CAD build for the part. Positions are in the model's coordinates, mm. Face numbers are marked on the shaded views. A direction names the side the tool comes from. Coordinates: 2 decimals unless noted, no trailing zeros. Loops run counter-clockwise (first coordinate to the right, second up) from the corner with the lowest first, then second, coordinate; pieces in that order, holes last. Notation, with made-up numbers: (20.25, -10.75) -> (56.25, -10.75) arc R17 ccw to (56.25, 3.25) -> close; hole circle Ø8 at (-22.75, 62). An arc over 180 degrees is marked (long way). Return JSON: item names as keys, results as strings. Group by question number.
(1) Saw through at B-B on y = 10.5. Write the cut outline in (x, z).
(2) Saw through at C-C on y = 5.25. Write the cut outline in (x, z), then the cut area to 3 significant figures.
(3) Flat gauge pins, fed straight in: pin 1 Ø4 at (x, y) = (-2, 14.5) entering from +Z; pin 2 Ø1.6 at (x, z) = (0, 0) entering from +Y; pin 3 Ø5 at (x, z) = (-2, 1.5) entering from +Y; pin 4 Ø4 at (y, z) = (18.5, 7.5) entering from +X. Where does each tip first touch, or does it go through?
(4) Tool access for the marked faces 1, 2 and 3: list every direction of +Z, -Z, +X, -X, +Y, -Y with a clear straight run to the whole face (end or side of a thin tool).
(5) Saw through at A-A on z = 0. Write the cut outline in (x, y), then the cut area to 3 significant figures.
(6) Probe L1, parallel to Z at x = 0, y = 3.85; L2, parallel to Z at x = 0, y = 11.5; L3, parallel to X at y = 0.35, z = 0. List the from-to ranges inside material, lowest first.
Autodesk Fusion 360 part; units mm, degrees
sketch "Sketch1" plane through (0, 0, 0) normal (0, 0, 1) x (1, 0, 0)
  line L0 (0, 0) -> (-8, 0)
  line L1 (-8, 0) -> (-8, 19)
  line L2 (-8, 19) -> (0, 19)
  line L3 (0, 19) -> (0, 0)
  line L4 (0, 19) -> (-6.75, 19)
  line L5 (-6.75, 19) -> (-6.75, 7)
  line L6 (-6.75, 7) -> (0, 7)
  line L7 (0, 7) -> (0, 19)
  line L8 (0, 7) -> (-3.5, 7)
  line L9 (-3.5, 7) -> (-3.5, 1)
  line L10 (-3.5, 1) -> (0, 1)
  line L11 (0, 1) -> (0, 7)
  line L12 (0, 19) -> (-11, 19)
  line L13 (-11, 19) -> (-11, 21)
  line L14 (-11, 21) -> (0, 21)
  line L15 (0, 21) -> (0, 19)
  line L16 (-6.75, 19) -> (-6.75, 21)
  line L17 (0, 1) -> (-1, 1)
  line L18 (-1, 1) -> (-1, 0)
  line L19 (-1, 0) -> (0, 0)
  line L20 (0, 0) -> (0, 1)
  dimension "d1" = 19
  dimension "d2" = 8
  dimension "d7" = 12
  dimension "d8" = 6.75
  dimension "d9" = 6
  dimension "d10" = 3.5
  dimension "d11" = 11
  dimension "d12" = 2
revolve "Revolve1" add sketch "Sketch1" angle 360 about axis through (0, 19, 0) along (0, -1, 0) contours L0 L1 L2 L5 L6 L9 L10 L12 L18 | L2 L12 L13 L14 L16
chamfer "Chamfer1" distance 1 angle 45 1 edges at (-10.2556, 21, 3.9778)
chamfer "Chamfer2" distance 0.5 angle 45 1 edges at (-6.2932, 21, 2.4409)
chamfer "Chamfer3" distance 2 angle 15 1 edges at (-6.2932, 7, 2.4409) measured on face at (-5.6285, 7, 0.5092)
chamfer "Chamfer4" distance 1 angle 30 1 edges at (-3.2631, 1, 1.2657) measured on face at (-2.6499, 1, 0.2236)
equation "d2 = Width / 2"
equation "Height = 19 mm"
equation "Width = 16 mm"
equation "LargeShank = 13.5 mm"
equation "SmallShank = 7 mm"
equation "d8 = LargeShank / 2"
equation "d10 = SmallShank / 2"
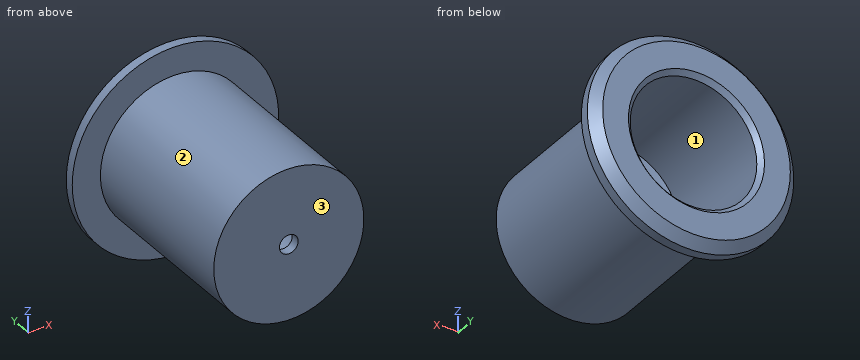
Geometry results:
{
 "1": {"outline": "circle Ø16 at (0, 0); hole circle Ø13.5 at (0, 0)"},
 "2": {"outline": "circle Ø16 at (0, 0); hole circle Ø7 at (0, 0)", "area": "163 mm²"},
 "3": {"pin 1": "z = 8", "pin 2": "through", "pin 3": "y = 7.07", "pin 4": "x = 9.49"},
 "4": {"face 1": "+Y", "face 2": "-Y", "face 3": "+Z, -Z, +X, -X, -Y"},
 "5": {"outline": "(-11, 19) -> (-8, 19) -> (-8, 0) -> (-1, 0) -> (-1, 1) -> (-2.5, 1) -> (-3.5, 1.58) -> (-3.5, 7) -> (-4.75, 7) -> (-6.75, 7.54) -> (-6.75, 20.5) -> (-7.25, 21) -> (-10, 21) -> (-11, 20) -> close; (1, 0) -> (8, 0) -> (8, 19) -> (11, 19) -> (11, 20) -> (10, 21) -> (7.25, 21) -> (6.75, 20.5) -> (6.75, 7.54) -> (4.75, 7) -> (3.5, 7) -> (3.5, 1.58) -> (2.5, 1) -> (1, 1) -> close", "area": "115 mm²"},
 "6": {"L1": "-8 to -3.5, 3.5 to 8", "L2": "-8 to -6.75, 6.75 to 8", "L3": "-8 to -1, 1 to 8"}
}
